Autodesk Fusion 360 part; units mm, degrees
sketch "Sketch1" plane through (0, 0, 0) normal (0, 1, 0) x (1, 0, 0)
  line L0 (-12, 40) -> (12, 40)
  line L1 (12, 40) -> (12, -40)
  line L2 (12, -40) -> (-12, -40)
  line L3 (-12, -40) -> (-12, 40)
  line L4 (-50, 0) -> (40, 0) construction
  line L5 (0, 60) -> (0, -56.3927) construction
  circle A0 centre (0, -28) radius 3.1
  circle A1 centre (0, 28) radius 3.1
  dimension "d1" = 24
  dimension "d2" = 80
  dimension "d3" = 12
  dimension "d4" = 40
  dimension "d5" = 6.2
  dimension "d6" = 12
  dimension "d7" = 12
extrude "Extrude1" add sketch "Sketch1" along normal blind 70
fillet "Fillet1" radius 3.5 4 edges at (-12, 35, 40) (-12, 35, -40) (12, 35, -40) (12, 35, 40)
sketch "Sketch3" plane through (12, 0, 0) normal (1, 0, 0) x (0, 0, -1)
  line L0 (-36.5, 70) -> (-36.5, 0)
  line L1 (-36.5, 0) -> (36.5, 0)
  line L2 (36.5, 0) -> (36.5, 70)
  line L3 (36.5, 70) -> (-36.5, 70)
  line L4 (36, 9) -> (-36, 9)
  line L5 (-36, 9) -> (-36, 61)
  line L6 (-36, 61) -> (36, 61)
  line L7 (36, 61) -> (36, 9)
  line L8 (36, 9) -> (-36, 61) construction
  line L9 (-36, 9) -> (36, 61) construction
  circle A0 centre (-36, 61) radius 1.25
  circle A1 centre (36, 61) radius 1.25
  circle A2 centre (-36, 9) radius 1.25
  circle A3 centre (36, 9) radius 1.25
  point P0 (0, 35)
  dimension "d12" = 72
  dimension "d13" = 52
  dimension "d14" = 36.5
  dimension "d15" = 73
  dimension "d16" = 2.5
  dimension "d17" = 2.5
  dimension "d18" = 2.5
  dimension "d19" = 2.5
  dimension "d20" = 70
  dimension "d21" = 35
extrude "Extrude2" cut sketch "Sketch3" against normal blind 24 contours L0 L5 L6 A0 | L0 A0 | L5 L6 A0 | L2 A1 | L2 L6 L7 A1 | L0 L4 L5 A2 | L0 A2 | L6 L7 A1 | L4 L5 A2 | L2 A3 | L2 L4 L7 A3 | L4 L7 A3
equation "d3 = d1 / 2"
equation "d4 = d2 / 2"
equation "d7 = d6"
equation "d14 = d15 / 2"
equation "d17 = d16"
equation "d18 = d16"
equation "d19 = d16"
equation "d21 = d20 / 2"
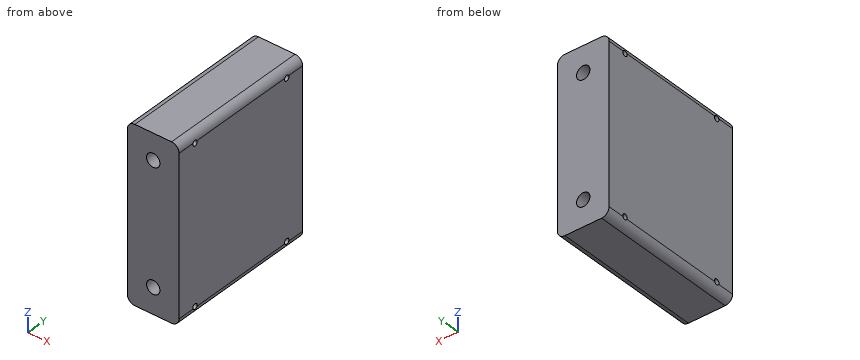
The model under review builds one solid part; all positions refer to its coordinate system, in mm. Round coordinates to 2 decimals unless told otherwise and drop trailing zeros. Loops run counter-clockwise (first coordinate to the right, second up) from the corner with the lowest first, then second, coordinate; pieces in that order, holes last. Notation, with made-up numbers: (-10.5, 31.25) - (4.5, 31.25) arc R20 ccw to (4.5, 54.25) - close; hole circle Ø9 at (12.5, 24.25). An arc over 180 degrees is marked (long way). Use CSV: the item, a comma, the result in double quotes.
(1) Take a section at B-B, the plane z = -28. Give the boundary of the cut face in (x, y).
Working result:
outline,"(-12, 0) - (-3.1, 0) - (-3.1, 70) - (-12, 70) - close; (3.1, 0) - (12, 0) - (12, 70) - (3.1, 70) - close"
(2) Clearance check with flat-ended pins moving along their axes: P1, Ø7, axis at x = 0, z = -28, coming from the -Y side; P2, Ø3.5, axis at x = 0, z = 28, coming from the +Y side. State where each tip first meets the part, or that it passes through.
Working result:
P1,"stops at y = 0"
P2,"passes through"
(3) Take a section at A-A, the plane x = 0. Give the boundary of the cut face in (y, z), plus the area to 3 significant figures.
Working result:
outline,"(0, -40) - (70, -40) - (70, -31.1) - (0, -31.1) - close; (0, -24.9) - (70, -24.9) - (70, 24.9) - (0, 24.9) - close; (0, 31.1) - (70, 31.1) - (70, 40) - (0, 40) - close; hole circle Ø2.5 at (9, -36); hole circle Ø2.5 at (9, 36); hole circle Ø2.5 at (61, -36); hole circle Ø2.5 at (61, 36)"
area,"4,710 mm^2"
(4) For line 1 (Z direction, x = -4.5, y = 61); line 2 (Y direction, x = 0.5, z = -36); line 3 (X direction, y = 43, z = -28), list the stretches that pass through material, from the lowest coordinate up.
Working result:
line 1,"z = -40 to -37.25, -34.75 to 34.75, 37.25 to 40"
line 2,"y = 0 to 7.75, 10.25 to 59.75, 62.25 to 70"
line 3,"x = -12 to -3.1, 3.1 to 12"
(5) Take a section at C-C, the plane y = 6. Give the boundary of the cut face in (x, z).
Working result:
outline,"(-12, -36.5) arc R3.5 ccw to (-8.5, -40) - (8.5, -40) arc R3.5 ccw to (12, -36.5) - (12, 36.5) arc R3.5 ccw to (8.5, 40) - (-8.5, 40) arc R3.5 ccw to (-12, 36.5) - close; hole circle Ø6.2 at (0, -28); hole circle Ø6.2 at (0, 28)"
